Could you check a few things on this drawing? It's one solid part, dimensions in mm from its lowest x, y, z. Give positions to 0.01 mm unless a question says otherwise; leave off trailing zeros. Loops run counter-clockwise (first coordinate to the right, second up) from the corner with the lowest first, then second, coordinate; pieces in that order, holes last. Notation, with made-up numbers: (26, 14) - (44, 14) arc R24 cw to (44, 31) - close; hole circle Ø11 at (-27.75, -22.75). An arc over 180 degrees is marked (long way). Use a Markdown table: item, result.
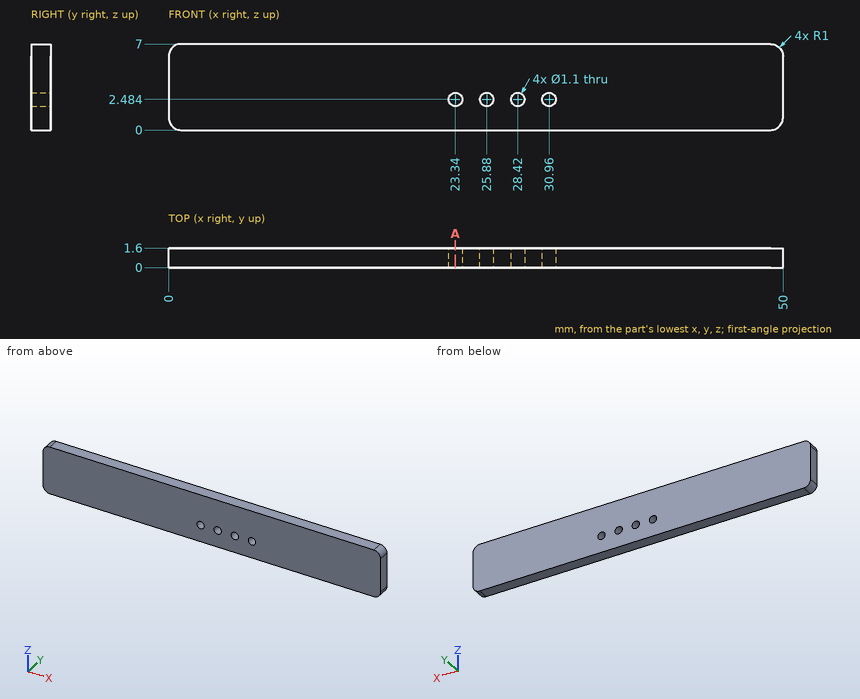
(1) Will this pin go through, and if not, where does the flat tip stop? pin 1 (0.9 mm diameter, centred on x = 25.88, z = 2.48, fed in from +Y).
A:
| item | result |
|---|---|
| pin 1 | through |
(2) If I drill on line 1 (X direction, y = 1.4, z = 2.5); line 2 (Z direction, x = 28.42, y = 1.2); line 3 (X direction, y = 0.7, z = 2.25), over which ranges is the centre line in solid material (lowest first)?
A:
| item | result |
|---|---|
| line 1 | 0 to 22.79, 23.89 to 25.33, 26.43 to 27.87, 28.97 to 30.41, 31.51 to 50 |
| line 2 | 0 to 1.93, 3.03 to 7 |
| line 3 | 0 to 22.84, 23.84 to 25.38, 26.38 to 27.92, 28.92 to 30.46, 31.46 to 50 |
(3) Suppose I cut it at A-A on x = 23.34. Write out the boundary of the cut face in (y, z).
A:
| item | result |
|---|---|
| outline | (0, 0) - (1.6, 0) - (1.6, 1.93) - (0, 1.93) - close; (0, 3.03) - (1.6, 3.03) - (1.6, 7) - (0, 7) - close |
